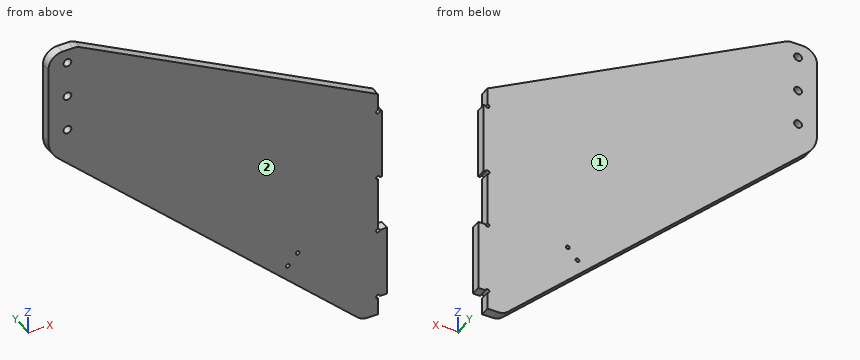
```python
from build123d import *

# Parameters (mm, degrees)
F0_R     = 2
F0_R_2   = 4.1
F1_DEPTH = 10
F2_R     = 30
F3_R     = 15


with BuildPart() as f1:
    # F0 (on Front) → F1 (new body)
    with BuildSketch(Plane.XZ):
        with BuildLine():
            Line((0, 310), (330, 0))
            Line((330, 0), (347, 0))
            Line((347, 0), (347, 18))
            ThreePointArc((347, 18), (345.585786, 21.414214), (349, 20))
            Line((349, 20), (356.5, 20))
            Line((356.5, 20), (356.5, 95))
            Line((356.5, 95), (349, 95))
            ThreePointArc((349, 95), (345.585786, 93.585786), (347, 97))
            Line((347, 97), (347, 153))
            ThreePointArc((347, 153), (345.585786, 156.414214), (349, 155))
            Line((349, 155), (351, 155))
            Line((351, 155), (351, 230))
            Line((351, 230), (349, 230))
            ThreePointArc((349, 230), (345.585786, 228.585786), (347, 232))
            Line((347, 232), (347, 250))
            Line((347, 250), (30, 420))
            Line((30, 420), (0, 420))
            Line((0, 420), (0, 310))
        make_face()
        with Locations((252.158545, 89.588128)):
            Circle(F0_R, mode=Mode.SUBTRACT)
        with Locations((262.428676, 100.520849)):
            Circle(F0_R, mode=Mode.SUBTRACT)
        with Locations((20, 329.4)):
            Circle(F0_R_2, mode=Mode.SUBTRACT)
        with Locations((20, 367.4)):
            Circle(F0_R_2, mode=Mode.SUBTRACT)
        with Locations((20, 405.4)):
            Circle(F0_R_2, mode=Mode.SUBTRACT)
    extrude(amount=F1_DEPTH)

    # F2
    f2_edges = [f1.edges().sort_by_distance(p)[0] for p in [
        (0, -5, 310),
    ]]
    fillet(f2_edges, radius=F2_R)

    # F3
    f3_edges = [f1.edges().sort_by_distance(p)[0] for p in [
        (0, -5, 420),
        (30, -5, 420),
        (330, -5, 0),
    ]]
    fillet(f3_edges, radius=F3_R)


solid = f1.part
```
Verification items for the finished model (mm, model axes). Face numbers are marked on the shaded views. Coordinates: 2 decimals unless noted, no trailing zeros. Order: outer loops, then holes, each group sorted by start corner. A loop starts at its lowest first (then second) coordinate and runs counter-clockwise, first axis right, second up. Notation, with made-up numbers: (-2.5, 64.5) -> (27.5, 64.5) arc R23 cw to (27.5, 75.5) -> close; hole circle Ø4 at (2, 57). An arc over 180 degrees is marked (long way). Put each result on its own line as item: value. Start each with the question number.
1) Go/stop test with flat-tipped pins: pin 1 (1.5 mm diameter, centred on x = 76.5, y = -6.5, fed in from -Z); pin 2 (5 mm diameter, centred on y = -5.5, z = 8, fed in from +X); pin 3 (3 mm diameter, centred on y = -7, z = 188, fed in from +X). Record where each tip stops, or that it passes through.
2) Material ranges on L1, parallel to Z at x = 20, y = -6.5; L2, parallel to Z at x = 220, y = -2; L3, parallel to Z at x = 40, y = -6.25, recorded low to high.
3) Cross-section at A-A (y = -5.5). Enter the section's corners in (x, z).
4) Release check for a two-part mould opening along Y. For the marked faces 1 and 2 record: pulls with the +Y half, pulls with the -Y half, needs draft (parallel to the pull), parting line crosses it, or undercut.
5) Cross-section at C-C (x = 107). Enter the section's corners in (y, z), plus the area to 3 significant figures.
6) Cross-section at B-B (z = 386). Enter the section's corners in (x, y).
Geometry check:
1. pin 1: stops at z = 237.43
1. pin 2: stops at x = 347
1. pin 3: stops at x = 351
2. L1: z = 291.21 to 325.3, 333.5 to 363.3, 371.5 to 401.3, 409.5 to 420
2. L2: z = 103.33 to 318.11
2. L3: z = 272.42 to 414.64
3. outline: (0, 322.98) arc R30 ccw to (9.46, 301.11) -> (325.67, 4.07) arc R15 ccw to (335.94, 0) -> (347, 0) -> (347, 18) arc R2 cw (long way) to (349, 20) -> (356.5, 20) -> (356.5, 95) -> (349, 95) arc R2 cw (long way) to (347, 97) -> (347, 153) arc R2 cw (long way) to (349, 155) -> (351, 155) -> (351, 230) -> (349, 230) arc R2 cw (long way) to (347, 232) -> (347, 250) -> (33.32, 418.22) arc R15 ccw to (26.23, 420) -> (15, 420) arc R15 ccw to (0, 405) -> close; hole circle Ø8.2 at (20, 329.4); hole circle Ø8.2 at (20, 367.4); hole circle Ø8.2 at (20, 405.4); hole circle Ø4 at (252.16, 89.59); hole circle Ø4 at (262.43, 100.52)
4. face 1: pulls with the +Y half
4. face 2: pulls with the -Y half
5. outline: (-10, 209.48) -> (0, 209.48) -> (0, 378.71) -> (-10, 378.71) -> close
5. area: 1,690 mm^2
6. outline: (0, -10) -> (93.4, -10) -> (93.4, 0) -> (0, 0) -> close
